from build123d import *

# Parameters (mm, degrees)
SKETCH1_R           = 14.5
SKETCH1_R_2         = 12.5
BOSS_EXTRUDE1_DEPTH = 11
SKETCH2_R           = 14.5
BOSS_EXTRUDE2_DEPTH = 1
SKETCH3_R           = 10.75
BOSS_EXTRUDE3_DEPTH = 15
SKETCH4_R           = 12.25
BOSS_EXTRUDE4_DEPTH = 11
FILLET1_R           = 0.5


with BuildPart() as part:
    # Sketch1 → Boss-Extrude1 (new body)
    with BuildSketch(Plane(origin=(0, 0, 0), x_dir=(1, 0, 0), z_dir=(0, 1, 0))):
        Circle(SKETCH1_R)
        Circle(SKETCH1_R_2, mode=Mode.SUBTRACT)
    extrude(amount=BOSS_EXTRUDE1_DEPTH)

    # Sketch2 → Boss-Extrude2 (add)
    with BuildSketch(Plane(origin=(0, 0, 0), x_dir=(-1, 0, 0), z_dir=(0, -1, 0))):
        Circle(SKETCH2_R)
    extrude(amount=BOSS_EXTRUDE2_DEPTH)

    # Sketch3 → Boss-Extrude3 (add)
    with BuildSketch(Plane.XZ.offset(1)):
        Circle(SKETCH3_R)
    extrude(amount=BOSS_EXTRUDE3_DEPTH)

    # Sketch4 → Boss-Extrude4 (add)
    with BuildSketch(Plane(origin=(0, 0, 0), x_dir=(1, 0, 0), z_dir=(0, 1, 0))):
        Circle(SKETCH4_R)
    extrude(amount=BOSS_EXTRUDE4_DEPTH)

    # Fillet1
    fillet1_edges = [part.edges().sort_by_distance(p)[0] for p in [
        (-12.25, 11, 0),
        (-14.5, 11, 0),
        (-12.5, 11, 0),
    ]]
    fillet(fillet1_edges, radius=FILLET1_R)


solid = part.part
The listing builds one solid part. Answer for the finished solid, in the listing's coordinates (mm). A direction names the side the tool comes from. Give positions to 0.01 mm unless a question says otherwise; leave off trailing zeros. Write each loop counter-clockwise with the first axis right and the second up, starting at its lowest first coordinate (ties: lowest second). Pieces come first, ordered by that corner, then holes.
1) Given P1, Ø6, axis at y = -7.5, z = 6.5, coming from the -X side; P2, Ø10, axis at y = 6.5, z = -5.5, coming from the +X side; P3, Ø4, axis at x = 7.5, y = -11.5, coming from the +Z side, each flat-ended and moving along its own axis, determine where each tip first touches the part or whether it passes through.
2) Find the intervals of material crossed by L1, parallel to Z at x = 0, y = 3; L2, parallel to Z at x = 9.75, y = 8.25, in increasing order.
3) For a pull along X with two mould halves and no side action, classify faces 1 (the face through (11.923, 5.176, -3.755)), 2 (the face through (-1.4, -8.4, 10.66)), 3 (the face through (9.3, 11, 9.3)), 4 (the face through (6.586, 5.176, -10.329)) as pulls with the +X half, pulls with the -X half, needs draft (parallel to the pull), parting line crosses it, or undercut.
4) Section B-B (x = 0) is taken. Write down the section's boundary in (y, z).
5) Section A-A (y = 5.5) is taken. Write down the section's boundary in (x, z).
6) Section C-C (z = 0) is taken. Write down the section's boundary in (x, y), and give its area (3 significant figures).
7) A tool of negligible diameter and unlimited length cuts with its end or side. For faces 5 (the face through (11, -1, 0)), 6 (the face through (0, 11, 0)), from which of +Z, -Z, +X, -X, +Y, -Y can it reach the whole face along a straight path? Write none if from no direction.
Response:
1. P1: stops at x = -10.16
1. P2: stops at x = 14.49
1. P3: stops at z = 9.24
2. L1: z = -14.5 to -12.5, -12.25 to 12.25, 12.5 to 14.5
2. L2: z = -10.73 to -7.82, -7.42 to 7.42, 7.82 to 10.73
3. face 1: undercut
3. face 2: parting line crosses it
3. face 3: needs draft
3. face 4: undercut
4. outline: (-16, -10.75) - (-1, -10.75) - (-1, -14.5) - (10.5, -14.5) arc R0.5 ccw to (11, -14) - (11, -13) arc R0.5 ccw to (10.5, -12.5) - (0, -12.5) - (0, -12.25) - (10.5, -12.25) arc R0.5 ccw to (11, -11.75) - (11, 11.75) arc R0.5 ccw to (10.5, 12.25) - (0, 12.25) - (0, 12.5) - (10.5, 12.5) arc R0.5 ccw to (11, 13) - (11, 14) arc R0.5 ccw to (10.5, 14.5) - (-1, 14.5) - (-1, 10.75) - (-16, 10.75) - close
5. outline: circle Ø29 at (0, 0); circle Ø24.5 at (0, 0); hole circle Ø25 at (0, 0)
6. outline: (-14.5, -1) - (-10.75, -1) - (-10.75, -16) - (10.75, -16) - (10.75, -1) - (14.5, -1) - (14.5, 10.5) arc R0.5 ccw to (14, 11) - (13, 11) arc R0.5 ccw to (12.5, 10.5) - (12.5, 0) - (12.25, 0) - (12.25, 10.5) arc R0.5 ccw to (11.75, 11) - (-11.75, 11) arc R0.5 ccw to (-12.25, 10.5) - (-12.25, 0) - (-12.5, 0) - (-12.5, 10.5) arc R0.5 ccw to (-13, 11) - (-14, 11) arc R0.5 ccw to (-14.5, 10.5) - close
6. area: 665 mm2
7. face 5: -Y
7. face 6: +Z, -Z, +X, -X, +Y
